from build123d import *

# Parameters (mm, degrees)
SKETCH1_W               = 25
SKETCH1_H               = 25
BOSS_EXTRUDE1_DEPTH     = 20
SKETCH2_R               = 14.5
CUT_EXTRUDE1_DEPTH      = 36.825056471
SKETCH3_W               = 6.310364348
SKETCH3_H               = 30
BOSS_EXTRUDE2_DEPTH     = 2
SKETCH4_W               = 10
SKETCH4_H               = 16
CUT_EXTRUDE2_DEPTH      = 30.497198662
CUT_EXTRUDE3_DEPTH      = 29.179509025
CUT_EXTRUDE3_DEPTH_BACK = 29.179509025
SKETCH5_R               = 1.75
SKETCH7_R               = 4.75
CUT_EXTRUDE4_DEPTH      = 29.179509089
CUT_SWEEP1_PROFILE_R    = 2
LPATTERN1_COUNT         = 2
LPATTERN1_PITCH         = 10
FILLET1_START           = -1
FILLET1_DEPTH           = 21
FILLET1_2_DEPTH         = 2
FILLET1_START_2         = 1.80548
FILLET1_3_DEPTH         = 18.19452
SKETCH11_W              = 2
SKETCH11_H              = 15
CUT_EXTRUDE5_DEPTH      = 38.652546889


with BuildPart() as part:
    # Sketch1 → Boss-Extrude1 (new body)
    with BuildSketch(Plane.XY):
        Rectangle(SKETCH1_W, SKETCH1_H)
    extrude(amount=BOSS_EXTRUDE1_DEPTH)

    # Sketch2 → Cut-Extrude1 (cut, through all)
    with BuildSketch(Plane(origin=(11.306356215, 0, -3.673657827), x_dir=(0, 1, 0), z_dir=(0.9510565162951534, 0, -0.3090169943749482))):
        with Locations((0, 25)):
            Circle(SKETCH2_R)
    extrude(amount=-CUT_EXTRUDE1_DEPTH, mode=Mode.SUBTRACT)

    # Sketch3 → Boss-Extrude2 (add)
    with BuildSketch(Plane.XY):
        with Locations((-12.5, 0)):
            Rectangle(SKETCH3_W, SKETCH3_H)
    extrude(amount=BOSS_EXTRUDE2_DEPTH)

    # Sketch4 → Cut-Extrude2 (cut, through all)
    with BuildSketch(Plane.XY):
        with Locations((-15.655182174, 0)):
            Rectangle(SKETCH4_W, SKETCH4_H)
    extrude(amount=CUT_EXTRUDE2_DEPTH, mode=Mode.SUBTRACT)

    # Sketch5 → Cut-Extrude3 (cut, two sides: drawn at the far end of the back side and taken through both)
    with BuildSketch(Plane.XY.offset(2).offset(-CUT_EXTRUDE3_DEPTH_BACK)):
        with Locations((-12, 11)):
            Circle(SKETCH5_R)
        with Locations((-12, -11)):
            Circle(SKETCH5_R)
    extrude(amount=CUT_EXTRUDE3_DEPTH + CUT_EXTRUDE3_DEPTH_BACK, mode=Mode.SUBTRACT)

    # Sketch7 → Cut-Extrude4 (cut, through all)
    with BuildSketch(Plane.XY.offset(2)):
        with Locations((-12, 11)):
            Circle(SKETCH7_R)
        with Locations((-12, -11)):
            Circle(SKETCH7_R)
    extrude(amount=CUT_EXTRUDE4_DEPTH, mode=Mode.SUBTRACT)

    # Cut-Sweep1: sweep along a path in Sketch8
    with BuildLine(Plane(origin=(1.795791052, 0, -0.583487883), x_dir=(0, 1, 0), z_dir=(0.9510565162951534, 0, -0.3090169943749482))) as cut_sweep1_path:
        CenterArc((0, 25), 18, 0, 360)
    # Cut-Sweep1 profile (on start of the path) → Cut-Sweep1 (sweep, cut)
    with BuildSketch(Plane(origin=(9.521215911, 18, 23.192925024), x_dir=(0.9510565162951534, 0, -0.3090169943749482), z_dir=(0.3090169943749482, 0, 0.9510565162951534))):
        Circle(CUT_SWEEP1_PROFILE_R)
    cut_sweep1 = sweep(path=cut_sweep1_path.line, mode=Mode.SUBTRACT)

    # LPattern1: Cut-Sweep1 ×2
    with Locations(*[Vector(-0.9510565162951534, 0, 0.3090169943749481) * (i * LPATTERN1_PITCH) for i in range(1, LPATTERN1_COUNT)]):
        add(cut_sweep1, mode=Mode.SUBTRACT)

    # Fillet1: read off the stored shape, not the designer's step
    # Fillet1 outline → Fillet1 (cut)
    with BuildSketch(Plane.XY.offset(FILLET1_START)):
        with BuildLine():
            ThreePointArc((-15.655182174, 13), (-15.069395736, 14.414213562), (-13.655182174, 15))
            Line((-13.655182174, 15), (-15.655182174, 15))
            Line((-15.655182174, 15), (-15.655182174, 13))
        make_face()
        with BuildLine():
            Line((-15.655182174, -15), (-13.655182174, -15))
            ThreePointArc((-13.655182174, -15), (-15.069395736, -14.414213562), (-15.655182174, -13))
            Line((-15.655182174, -13), (-15.655182174, -15))
        make_face()
    extrude(amount=FILLET1_DEPTH, mode=Mode.SUBTRACT)

    # Fillet1 2 outline → Fillet1 2 (add)
    with BuildSketch(Plane.XY):
        with BuildLine():
            Line((-9.344817826, 14.5), (-9.344817826, 12.5))
            Line((-9.344817826, 12.5), (-7.344817826, 12.5))
            ThreePointArc((-7.344817826, 12.5), (-8.759031388, 13.085786438), (-9.344817826, 14.5))
        make_face()
        with BuildLine():
            Line((-9.344817826, -12.5), (-9.344817826, -14.5))
            ThreePointArc((-9.344817826, -14.5), (-8.759031388, -13.085786438), (-7.344817826, -12.5))
            Line((-7.344817826, -12.5), (-9.344817826, -12.5))
        make_face()
    extrude(amount=FILLET1_2_DEPTH)

    # Fillet1 3 outline → Fillet1 3 (add)
    with BuildSketch(Plane.XY.offset(FILLET1_START_2)):
        with BuildLine():
            ThreePointArc((-7.344817826, 12.5), (-7.419933265, 12.50141108), (-7.494942711, 12.505642329))
            ThreePointArc((-7.494942711, 12.505642329), (-7.494000925, 12.502821459), (-7.493060906, 12.5))
            Line((-7.493060906, 12.5), (-7.344817826, 12.5))
        make_face()
        with BuildLine():
            ThreePointArc((-7.493060906, -12.5), (-7.494000925, -12.502821459), (-7.494942711, -12.505642329))
            ThreePointArc((-7.494942711, -12.505642329), (-7.419933265, -12.50141108), (-7.344817826, -12.5))
            Line((-7.344817826, -12.5), (-7.493060906, -12.5))
        make_face()
    extrude(amount=FILLET1_3_DEPTH)

    # Sketch11 → Cut-Extrude5 (cut, through all)
    with BuildSketch(Plane(origin=(12.5, 0, 0), x_dir=(0, 0, -1), z_dir=(1, 0, 0))):
        Rectangle(SKETCH11_W, SKETCH11_H)
    extrude(amount=-CUT_EXTRUDE5_DEPTH, mode=Mode.SUBTRACT)


solid = part.part
Read the model definition and answer for the solid it produces. Units are mm, in the model's axes. A direction names the side the tool comes from. Coordinates: 2 decimals unless noted, no trailing zeros. Loops run counter-clockwise (first coordinate to the right, second up) from the corner with the lowest first, then second, coordinate; pieces in that order, holes last.
Q1. Which of the six approach directions +Z, -Z, +X, -X, +Y, -Y give full straight-line access (tool end or side, diameter ignored) to faces 1 (the face through (-13, -8, 1)), 2 (the face through (-7.765, -8.849, 8.874)), 3 (the face through (1.1, 7.5, 0.5))?
Q2. Each of these flat-tipped pins is pushed along its axis until it touches: pin 1 Ø4.5 at (x, y) = (-12, -11) entering from -Z; pin 2 Ø5 at (y, z) = (3, 7) entering from -X; pin 3 Ø6 at (x, z) = (1.5, 9.5) entering from +Y; pin 4 Ø12 at (x, y) = (0.5, 1) entering from -Z. Where does it stop, or does it pass through?
Q3. The mould has two halves that part along Y. Classify faces 4 (the face through (-11.1, 12.5, 1)), 5 (the face through (1.1, -7.5, 0.5)), 6 (the face through (-15.655, -11, 1)), 7 (the face through (-15.054, -14.43, 0.986)): +Y half, -Y half, draft (parallel to the pull), parting line (faces both ways), or undercut.
Q4. The part is cut by section B-B on y = 11. Give the number of separate pieces and of enclosed holes in the cut face, and give its area (3 significant figures).
Q5. The part is cut by section A-A on x = -12. Write down the section's boundary in (y, z), and give its area (3 significant figures).
Q6. Consider probe 1 along Y at (x, z) = (-12, 1.45); probe 2 along X at (y, z) = (11, 1.1); probe 3 along X at (y, z) = (-0.5, 3). Determine where each line is inside the solid, lowest interval first.
Results below:
1. face 1: +Z, -Z, -X
1. face 2: +Z, -X
1. face 3: -Z, +X, -X
2. pin 1: stops at z = 0
2. pin 2: stops at x = -10.66
2. pin 3: stops at y = 12.5
2. pin 4: stops at z = 1
3. face 4: undercut
3. face 5: undercut
3. face 6: draft
3. face 7: -Y half
4. separate pieces: 2
4. enclosed holes: 2
4. area: 284 mm2
5. outline: (-15, 0) - (-12.75, 0) - (-12.75, 2) - (-15, 2) - close; (-9.25, 0) - (-8, 0) - (-8, 2) - (-9.25, 2) - close; (8, 0) - (9.25, 0) - (9.25, 2) - (8, 2) - close; (12.75, 0) - (15, 0) - (15, 2) - (12.75, 2) - close
5. area: 14.0 mm2
6. probe 1: y = -15 to -12.75, -9.25 to -8, 8 to 9.25, 12.75 to 15
6. probe 2: x = -15.66 to -13.75, -10.25 to 12.5
6. probe 3: x = -10.66 to 12.5
